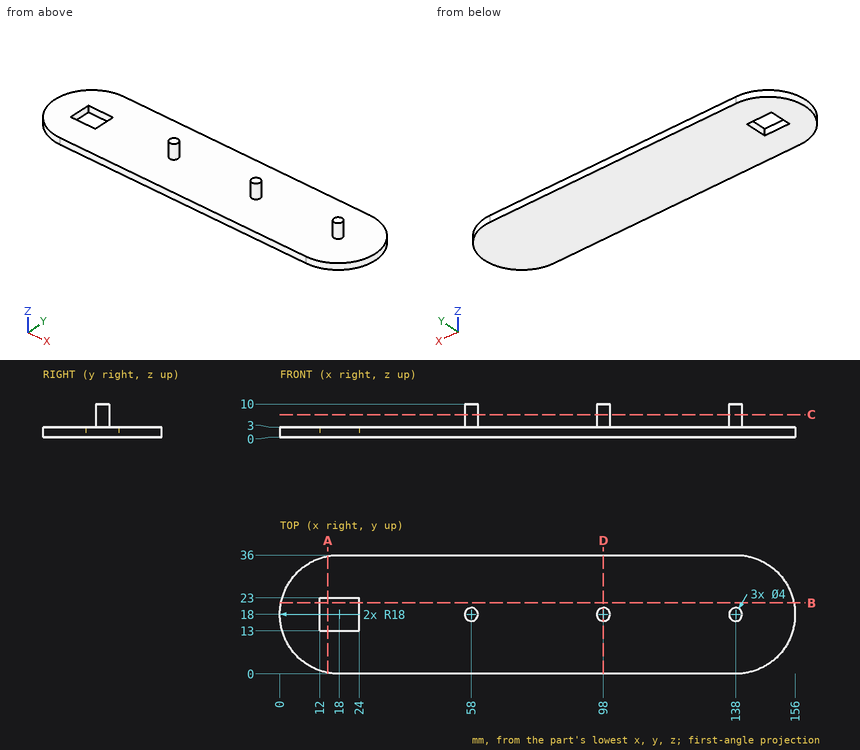
Source: three-view drawing plus pictorial views. Frame: mm from the lowest corner of the part. Round coordinates to 2 decimals unless told otherwise and drop trailing zeros. Write each loop counter-clockwise with the first axis right and the second up, starting at its lowest first coordinate (ties: lowest second). Pieces come first, ordered by that corner, then holes. Notation, with made-up numbers: M -6.5,27 L 50.5,27 A21 ccw 50.5,58 Z; hole C 34.5,44 d10. An arc over 180 degrees is marked long. One line per item, written item: value. Start each with the question number.
Item 1: Section query D-D (x = 98). Return the cut outline in (y, z), plus the area to 3 significant figures.
Item 2: Section query B-B (y = 21.5). Return the cut outline in (x, z), plus the area to 3 significant figures.
Item 3: Section query A-A (x = 14.5). Return the cut outline in (y, z), plus the area to 3 significant figures.
Item 4: Ray query, L1, parallel to Z at x = 138, y = 4; L2, parallel to Y at x = 98, z = 4.5; L3, parallel to Y at x = 57.5, z = 8.25. Return the intervals inside material, ascending. Write a range as from..to.
Item 5: Section query C-C (z = 6.75). Return the cut outline in (x, y).
Item 6: Pin query (flat end, axial travel): pin 1 (2 mm diameter, centred on x = 31.5, y = 31.5, fed in from +Z); pin 2 (2 mm diameter, centred on x = 83.5, y = 19, fed in from -Z); pin 3 (1.5 mm diameter, centred on x = 16, z = 1.5, fed in from +Y); pin 4 (0.9 mm diameter, centred on y = 18, z = 2, fed in from +X). Return the tip coordinate at first contact, or that it passes through.
Result set:
1. outline: M 0,0 L 36,0 L 36,3 L 20,3 L 20,10 L 16,10 L 16,3 L 0,3 Z
1. area: 136 mm²
2. outline: M 0.34,0 L 12,0 L 12,3 L 0.34,3 Z; M 24,0 L 155.66,0 L 155.66,3 L 24,3 Z
2. area: 430 mm²
3. outline: M 0.34,0 L 13,0 L 13,3 L 0.34,3 Z; M 23,0 L 35.66,0 L 35.66,3 L 23,3 Z
3. area: 75.9 mm²
4. L1: z = 0..3
4. L2: y = 16..20
4. L3: y = 16.06..19.94
5. outline: C 58,18 d4; C 98,18 d4; C 138,18 d4
6. pin 1: stops at z = 3
6. pin 2: stops at z = 0
6. pin 3: stops at y = 35.96
6. pin 4: stops at x = 156
